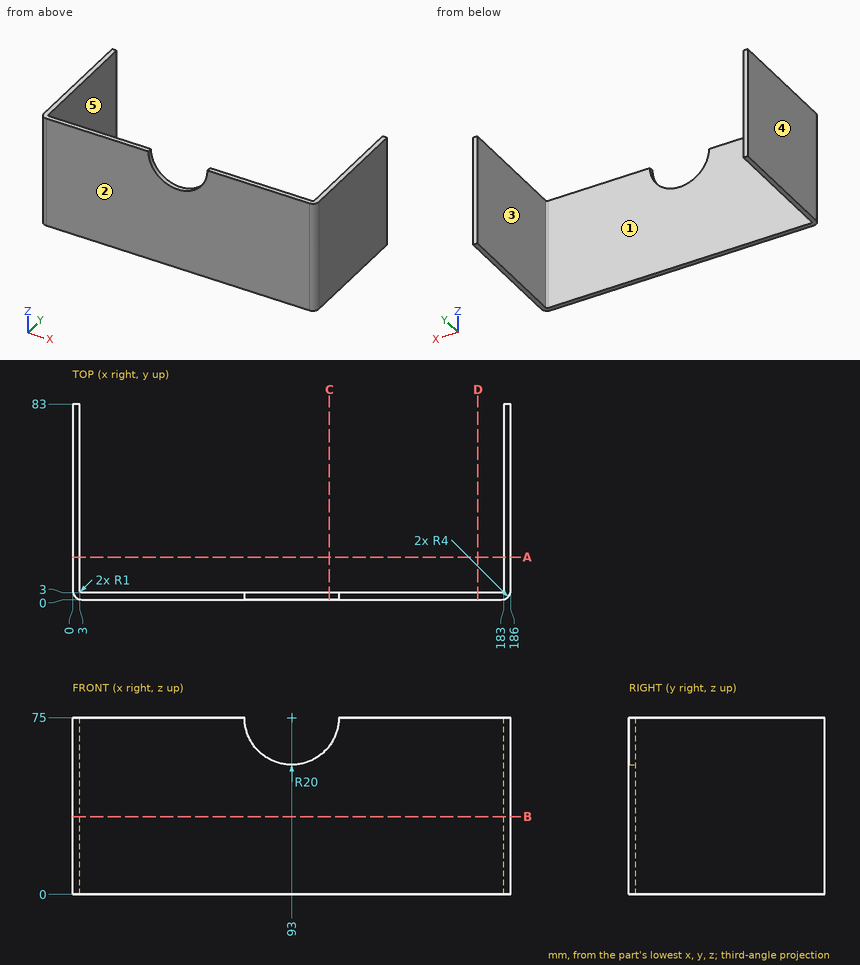
Part print with two shaded views. Sizes in mm from the minimum x, y, z corner. A direction names the side the tool comes from. Round coordinates to 2 decimals unless told otherwise and drop trailing zeros. Order: outer loops, then holes, each group sorted by start corner. A loop starts at its lowest first (then second) coordinate and runs counter-clockwise, first axis right, second up. Notation, with made-up numbers: (58.5, 1) - (74.5, 1) arc R13 cw to (74.5, 14) - close; hole circle Ø9 at (26, 12.25). An arc over 180 degrees is marked (long way). Return JSON: item names as keys, results as strings.
(1) Pin check, flat tip, straight feed: pin 1 Ø2 at (x, z) = (43.5, 64.5) entering from +Y. Stop position of the tip, or through.
Answer key:
{"pin 1": "stops at y = 3"}
(2) Cut at B-B (z = 33). Give the cut face in (x, y).
Answer key:
{"outline": "(0, 4) arc R4 ccw to (4, 0) - (182, 0) arc R4 ccw to (186, 4) - (186, 83) - (183, 83) - (183, 4) arc R1 cw to (182, 3) - (4, 3) arc R1 cw to (3, 4) - (3, 83) - (0, 83) - close"}
(3) Tool access for the marked faces 4 and 5: list every direction of +Z, -Z, +X, -X, +Y, -Y with a clear straight run to the whole face (end or side of a thin tool).
Answer key:
{"face 4": "+Z, -Z, -X, +Y, -Y", "face 5": "+Z, -Z, +Y"}
(4) Pull direction Y, two halves, no side cores. Call the marked faces 1, 2 and 3: +Y half, -Y half, draft (parallel to the pull), parting line (faces both ways), or undercut.
Answer key:
{"face 1": "+Y half", "face 2": "-Y half", "face 3": "draft"}
(5) Cut at A-A (y = 18). Give the cut face in (x, z), then the cut area to 3 significant figures.
Answer key:
{"outline": "(0, 0) - (3, 0) - (3, 75) - (0, 75) - close; (183, 0) - (186, 0) - (186, 75) - (183, 75) - close", "area": "450 mm^2"}
(6) Wall check: probe 1 along X at (y, z) = (9, 13); probe 2 along Y at (x, z) = (152.5, 62.5). Give the ranges that are in metal, low to high. Write a range as from..to.
Answer key:
{"probe 1": "x = 0..3, 183..186", "probe 2": "y = 0..3"}
(7) Cut at D-D (x = 172). Give the cut face in (y, z), then the cut area to 3 significant figures.
Answer key:
{"outline": "(0, 0) - (3, 0) - (3, 75) - (0, 75) - close", "area": "225 mm^2"}
(8) Cut at C-C (x = 109). Give the cut face in (y, z), then the cut area to 3 significant figures.
Answer key:
{"outline": "(0, 0) - (3, 0) - (3, 63) - (0, 63) - close", "area": "189 mm^2"}
